Autodesk Inventor part; units mm, degrees
ref_plane "YZ Plane" through (0, 0, 0) normal (1, 0, 0) x (0, 1, 0)
ref_plane "XZ Plane" through (0, 0, 0) normal (0, 1, 0) x (-1, 0, 0)
ref_plane "XY Plane" through (0, 0, 0) normal (0, 0, 1) x (1, 0, 0)
sketch "Sketch1" plane through (0, 0, 0) normal (0, 0, 1) x (1, 0, 0)
  line L0 (-30, 0) -> (30, 0)
  line L1 (30, 0) -> (30, 20)
  line L2 (30, 20) -> (10, 60)
  line L3 (10, 60) -> (-10, 60)
  line L4 (-10, 60) -> (-30, 20)
  line L5 (-30, 20) -> (-30, 0)
  circle A0 centre (0, 50) radius 2.75
  circle A1 centre (0, 30) radius 2.75
  circle A2 centre (20, 10) radius 2.75
  circle A3 centre (-20, 10) radius 2.75
  point P0 (0, 0)
  point P1 (0, 0)
  point P2 (0, 60)
  dimension "d0" = 60
  dimension "d1" = 60
  dimension "d2" = 20
  dimension "d3" = 20
  dimension "d4" = 5.5
  dimension "d5" = 10
  dimension "d6" = 20
  dimension "d7" = 10
  dimension "d8" = 10
  dimension "d9" = 10
extrude "Extrusion1" add sketch "Sketch1" along normal blind 5
properties part number "SupportCR-10-Mini"
CAD build for the part. Positions are in the model's coordinates, mm. Coordinates: 2 decimals unless noted, no trailing zeros. Order: outer loops, then holes, each group sorted by start corner. A loop starts at its lowest first (then second) coordinate and runs counter-clockwise, first axis right, second up.
(1) Saw through at D-D, the plane y = 50. Write the cut outline in (x, z).
Solution:
outline: (-15, 0) - (-2.75, 0) - (-2.75, 5) - (-15, 5) - close; (2.75, 0) - (15, 0) - (15, 5) - (2.75, 5) - close
(2) Saw through at C-C, the plane x = 20. Write the cut outline in (y, z), and give its area (4 significant figures).
Solution:
outline: (0, 0) - (7.25, 0) - (7.25, 5) - (0, 5) - close; (12.75, 0) - (40, 0) - (40, 5) - (12.75, 5) - close
area: 172.5 mm2
(3) Saw through at B-B, the plane y = 10. Write the cut outline in (x, z).
Solution:
outline: (-30, 0) - (-22.75, 0) - (-22.75, 5) - (-30, 5) - close; (-17.25, 0) - (17.25, 0) - (17.25, 5) - (-17.25, 5) - close; (22.75, 0) - (30, 0) - (30, 5) - (22.75, 5) - close
(4) Drill centre lines: L1, parallel to X at y = 11, z = 2.1; L2, parallel to X at y = 12, z = 2; L3, parallel to Y at x = 1, z = 4.55. Where is each one in solid material? Low to high.
Solution:
L1: x = -30 to -22.56, -17.44 to 17.44, 22.56 to 30
L2: x = -30 to -21.89, -18.11 to 18.11, 21.89 to 30
L3: y = 0 to 27.44, 32.56 to 47.44, 52.56 to 60
(5) Saw through at A-A, the plane x = 0. Write the cut outline in (y, z).
Solution:
outline: (0, 0) - (27.25, 0) - (27.25, 5) - (0, 5) - close; (32.75, 0) - (47.25, 0) - (47.25, 5) - (32.75, 5) - close; (52.75, 0) - (60, 0) - (60, 5) - (52.75, 5) - close
(6) Pin check, flat tips, straight feed: pin 1 Ø5 at (x, y) = (-20, 10) entering from +Z; pin 2 Ø3 at (x, z) = (-17.5, 0.5) entering from +Y; pin 3 Ø2 at (y, z) = (23.5, 4.5) entering from +X; pin 4 Ø1 at (x, z) = (15.5, 1.5) entering from +Y. Stop position of each tip, or through.
Solution:
pin 1: passes through
pin 2: stops at y = 48
pin 3: stops at x = 28.75
pin 4: stops at y = 50
(7) Mould opens along X. For faces 1 (the face through (-20, 40, 2)), 2 (the face through (0, 24, 5)), 3 (the face through (17.253, 9.879, 2.465)), 4 (the face through (-22.747, 9.879, 2.465)) say: released by +X, released by -X, zero draft, split by the parting line, or undercut.
Solution:
face 1: released by -X
face 2: zero draft
face 3: undercut
face 4: undercut
